Autodesk Inventor part; units mm, degrees
ref_plane "Work Plane3" through (16.78, -11.54, 5.4873) normal (0, 0, -1) x (0, 1, 0)
ref_plane "Work Plane4" through (20.4057, 11.4343, 2.7437) normal (0, 0, 1) x (1, 0, 0)
ref_plane "YZ Plane" through (0, 0, 0) normal (1, 0, 0) x (0, 1, 0)
sketch "Sketch4" plane through (0, 0, 0) normal (0, 0, 1) x (1, 0, 0)
  circle A0 centre (49.58, 12.36) radius 1.25
  circle A1 centre (49.58, -8.84) radius 1.25
  line L0 (43.38, -11.54) -> (43.38, 15.06)
  line L1 (43.38, 15.06) -> (16.78, 15.06)
  line L2 (16.78, 15.06) -> (16.78, -11.54)
  line L3 (16.78, -11.54) -> (43.38, -11.54)
  line L4 (41.7543, -9.9143) -> (18.4057, -9.9143)
  line L5 (18.4057, -9.9143) -> (18.4057, 13.4343)
  line L6 (18.4057, 13.4343) -> (41.7543, 13.4343)
  line L7 (41.7543, 13.4343) -> (41.7543, -9.9143)
  circle A2 centre (20.4057, 11.4343) radius 2
  circle A3 centre (49.58, 12.36) radius 2.5
  point P0 (0, 0)
  dimension "d8" = 4
  dimension "d9" = 5
ref_plane "Work Plane3" through (16.78, -11.54, 5.4873) normal (0, 0, -1) x (0, 1, 0)
extrude "Extrusion3" add sketch "Sketch4" along normal up to surface (5.4873 mm away) contours A0 | A2 | A3
ref_plane "Work Plane4" through (20.4057, 11.4343, 2.7437) normal (0, 0, 1) x (1, 0, 0)
sketch "Sketch5" plane through (20.4057, 11.4343, 2.7437) normal (0, 0, 1) x (1, 0, 0)
  circle A0 centre (0, 0) radius 2
  circle A1 centre (29.1743, 0.9257) radius 2.5
  line L0 (-0.0977, 1.9976) -> (29.0523, 3.4227)
  circle A2 centre (29.1743, 0.9257) radius 2.5
  line L1 (29.2108, -1.5741) -> (0.0292, -1.9998)
  point P0 (-20.4057, -11.4343)
  point P1 (29.0523, 3.4227)
extrude "Extrusion4" add sketch "Sketch5" along normal mid plane 2 contours A0 L0 A1 L1
sketch "Sketch6" plane through (49.58, 12.36, 0) normal (0, 0, -1) x (-1, 0, 0)
  circle A0 centre (0, 0) radius 2.5
  point P0 (49.58, -12.36)
hole "Hole1" at (49.58, 12.36, 0) direction (0, 0, 1) diameter 2.013 end through all
properties part number "DualPMTController.ScreenSpacer"
Work out the finished part from the listing and answer in its coordinate system (mm). A direction names the side the tool comes from. Round coordinates to 2 decimals unless told otherwise and drop trailing zeros. Write each loop counter-clockwise with the first axis right and the second up, starting at its lowest first coordinate (ties: lowest second). Pieces come first, ordered by that corner, then holes.
1) A cutting plane is placed at C-C on y = 10.95. Determine the outline of the cut face in (x, z).
2) A cutting plane is placed at A-A on y = 12.36. Determine the outline of the cut face in (x, z).
3) A cutting plane is placed at D-D on z = 2.1. Determine the outline of the cut face in (x, y).
4) Which of the six approach directions +Z, -Z, +X, -X, +Y, -Y give full straight-line access (tool end or side, diameter ignored) to faces 4 (the face through (20, 11, 0)), 5 (the face through (51.89, 13.32, 2.71))?
5) Consider probe 1 along Y at (x, z) = (49.58, 1.4); probe 2 along X at (y, z) = (12.36, 1.35); probe 3 along X at (y, z) = (12.55, 5). Determine where each line is inside the solid, lowest interval first.
6) Determine the mould class of faces 1 (the face through (34.679, 14.134, 2.73)), 2 (the face through (50, 11, 0)), 3 (the face through (50.473, 12.824, 2.782)) for opening direction Y: pulls with the +Y half, pulls with the -Y half, needs draft (parallel to the pull), parting line crosses it, or undercut.
7) Flat-ended cylindrical pins translate along their axes: P1, Ø1.5, axis at x = 31.5, y = 13, coming from the -Z side; P2, Ø2, axis at x = 41, y = 12, coming from the +Z side; P3, Ø1.6, axis at x = 49.58, y = 12.36, coming from the +Z side; P4, Ø1, axis at x = 44, z = 3, coming from the +Y side. Find the tip coordinate at first contact, or state that the pin passes through.
8) A cutting plane is placed at B-B on z = 5. Determine the outline of the cut face in (x, y), and give its area (3 significant figures).
Entries:
1. outline: (18.47, 0) - (22.35, 0) - (22.35, 1.74) - (47.52, 1.74) - (47.52, 0) - (51.64, 0) - (51.64, 5.49) - (47.52, 5.49) - (47.52, 3.74) - (22.35, 3.74) - (22.35, 5.49) - (18.47, 5.49) - close
2. outline: (18.63, 0) - (22.18, 0) - (22.18, 1.74) - (47.08, 1.74) - (47.08, 0) - (48.57, 0) - (48.57, 5.49) - (47.08, 5.49) - (47.08, 3.74) - (22.18, 3.74) - (22.18, 5.49) - (18.63, 5.49) - close; (50.59, 0) - (52.08, 0) - (52.08, 5.49) - (50.59, 5.49) - close
3. outline: (20.31, 13.43) arc R2 ccw to (20.43, 9.43) - (49.62, 9.86) arc R2.5 ccw (long way) to (49.46, 14.86) - close; hole circle Ø2.01 at (49.58, 12.36)
4. face 4: -Z, +X, -X, +Y, -Y
4. face 5: none
5. probe 1: y = 9.86 to 11.35, 13.37 to 14.86
5. probe 2: x = 18.63 to 22.18, 47.08 to 48.57, 50.59 to 52.08
5. probe 3: x = 18.75 to 22.07, 47.09 to 48.59, 50.57 to 52.07
6. face 1: pulls with the +Y half
6. face 2: needs draft
6. face 3: undercut
7. P1: stops at z = 1.74
7. P2: stops at z = 3.74
7. P3: passes through
7. P4: stops at y = 14.61
8. outline: circle Ø4 at (20.41, 11.43); circle Ø5 at (49.58, 12.36); hole circle Ø2.01 at (49.58, 12.36)
8. area: 29.0 mm2
